Input: part model. Units: mm. Frame: model coordinates. A direction names the side the tool comes from. Coordinates: 2 decimals unless noted, no trailing zeros. Write each loop counter-clockwise with the first axis right and the second up, starting at its lowest first coordinate (ties: lowest second). Pieces come first, ordered by that corner, then holes.
1) Section query B-B (x = 0). Output: boundary loops of the cut face in (y, z), then the cut area to 3 significant figures.
2) Section query D-D (x = 3.5). Output: boundary loops of the cut face in (y, z).
3) Line query: L1, parallel to X at y = -2, z = 8; L2, parallel to X at y = -0.5, z = 6.25; L3, parallel to Y at x = -5, z = 2.5. Output: solid intervals per line, ascending.
4) Section query A-A (z = 5.25). Output: boundary loops of the cut face in (x, y).
5) Pin query (flat end, axial travel): pin 1 Ø1.5 at (x, y) = (1.5, -3) entering from -Z; pin 2 Ø3 at (x, y) = (12.5, 0.5) entering from +Z. Return the tip coordinate at first contact, or that it passes through.
6) Section query C-C (y = -2). Output: boundary loops of the cut face in (x, z), then the cut area to 3 significant figures.
7) Set-up query: faces 4 (the cylindrical face through (5.119, -2.175, -0.877)), 5 (the flat face through (0, 2.68, 6)), 6 (the flat face through (-8, 0, 9.601)). Return all of +Z, -Z, +X, -X, +Y, -Y with unobstructed straight access to the full face (end or side cutting, diameter ignored); none if empty.
8) Draft query along X for faces 1 (the flat face through (15.913, 0, 5)), 2 (the flat face through (8, 0, 9.601)), 3 (the flat face through (0, 0, 0)). Return one class per face: pulls with the +X half, pulls with the -X half, needs draft (parallel to the pull), parting line crosses it, or undercut.
from build123d import *

# Parameters (mm, degrees)
F0_W     = 31.8262
F0_H     = 7.8486
F2_DEPTH = 9.6012
F1_R     = 2.4511
F3_DEPTH = 1.778
F4_W     = 29.337
F4_H     = 5.3594
F6_DEPTH = 7.62
F5_R     = 1.4859
F7_DEPTH = 8.128


with BuildPart() as f2:
    # F0 (on Top) → F2 (new body)
    with BuildSketch(Plane.XY):
        Rectangle(F0_W, F0_H)
    extrude(amount=F2_DEPTH)

    # F1 (on face) → F3 (join)
    with BuildSketch(Plane.XY):
        with Locations((-11.9634, 0)):
            Circle(F1_R)
        with Locations((-3.9878, 0)):
            Circle(F1_R)
        with Locations((3.9878, 0)):
            Circle(F1_R)
        with Locations((11.9634, 0)):
            Circle(F1_R)
    extrude(amount=-F3_DEPTH)

    # F4 (on face) → F6 (cut)
    with BuildSketch(Plane.XY.offset(9.6012)):
        Rectangle(F4_W, F4_H)
    extrude(amount=-F6_DEPTH, mode=Mode.SUBTRACT)

    # F5 (on face) → F7 (join)
    with BuildSketch(Plane.XY.offset(9.6012)):
        with Locations((-7.9756, 0)):
            Circle(F5_R)
        Circle(F5_R)
        with Locations((7.9756, 0)):
            Circle(F5_R)
    extrude(amount=-F7_DEPTH)


solid = f2.part
Answer:
1. outline: (-3.92, 0) - (3.92, 0) - (3.92, 9.6) - (2.68, 9.6) - (2.68, 1.98) - (1.49, 1.98) - (1.49, 9.6) - (-1.49, 9.6) - (-1.49, 1.98) - (-2.68, 1.98) - (-2.68, 9.6) - (-3.92, 9.6) - close
1. area: 57.2 mm2
2. outline: (-3.92, 0) - (-2.4, 0) - (-2.4, -1.78) - (2.4, -1.78) - (2.4, 0) - (3.92, 0) - (3.92, 9.6) - (2.68, 9.6) - (2.68, 1.98) - (-2.68, 1.98) - (-2.68, 9.6) - (-3.92, 9.6) - close
3. L1: x = -15.91 to -14.67, 14.67 to 15.91
3. L2: x = -15.91 to -14.67, -9.37 to -6.58, -1.4 to 1.4, 6.58 to 9.37, 14.67 to 15.91
3. L3: y = -3.92 to -2.68, 2.68 to 3.92
4. outline: (-15.91, -3.92) - (15.91, -3.92) - (15.91, 3.92) - (-15.91, 3.92) - close; circle Ø2.97 at (-7.98, 0); circle Ø2.97 at (0, 0); circle Ø2.97 at (7.98, 0); hole (-14.67, -2.68) - (14.67, -2.68) - (14.67, 2.68) - (-14.67, 2.68) - close
5. pin 1: stops at z = 0
5. pin 2: stops at z = 1.98
6. outline: (-15.91, 0) - (-13.38, 0) - (-13.38, -1.78) - (-10.55, -1.78) - (-10.55, 0) - (-5.4, 0) - (-5.4, -1.78) - (-2.57, -1.78) - (-2.57, 0) - (2.57, 0) - (2.57, -1.78) - (5.4, -1.78) - (5.4, 0) - (10.55, 0) - (10.55, -1.78) - (13.38, -1.78) - (13.38, 0) - (15.91, 0) - (15.91, 9.6) - (14.67, 9.6) - (14.67, 1.98) - (-14.67, 1.98) - (-14.67, 9.6) - (-15.91, 9.6) - close
6. area: 102 mm2
7. face 4: -Z
7. face 5: +Z
7. face 6: +Z, +X, -X, +Y, -Y
8. face 1: pulls with the +X half
8. face 2: needs draft
8. face 3: undercut
